from build123d import *

# Parameters (mm, degrees)
SKETCH1_R           = 1.5
BOSS_EXTRUDE1_DEPTH = 3


with BuildPart() as part:
    # Sketch1 → Boss-Extrude1 (new body)
    with BuildSketch(Plane.XY):
        with BuildLine():
            ThreePointArc((-0.4997558, 7.984375), (-0.738146876, 7.96587341), (-0.975878549, 7.94025573))
            ThreePointArc((-0.975878549, 7.94025573), (-1.378121384, 7.372298248), (-1.958371564, 7.756595956))
            ThreePointArc((-1.958371564, 7.756595956), (-2.189303921, 7.694605145), (-2.418280524, 7.625740574))
            ThreePointArc((-2.418280524, 7.625740574), (-2.709312496, 6.993541721), (-3.350297333, 7.264675339))
            ThreePointArc((-3.350297333, 7.264675339), (-3.565906846, 7.161306331), (-3.778330856, 7.05153997))
            ThreePointArc((-3.778330856, 7.05153997), (-3.948241222, 6.376628518), (-4.628132745, 6.525364917))
            ThreePointArc((-4.628132745, 6.525364917), (-4.821077091, 6.384137818), (-5.009714662, 6.237207629))
            ThreePointArc((-5.009714662, 6.237207629), (-5.052717327, 5.542566879), (-5.748362647, 5.563841018))
            ThreePointArc((-5.748362647, 5.563841018), (-5.912071338, 5.389565149), (-6.070498644, 5.210474662))
            ThreePointArc((-6.070498644, 5.210474662), (-5.985129205, 4.519759773), (-6.672838954, 4.412847187))
            ThreePointArc((-6.672838954, 4.412847187), (-6.801737086, 4.211457303), (-6.924559076, 4.006305231))
            ThreePointArc((-6.924559076, 4.006305231), (-6.713724685, 3.343037668), (-7.370079733, 3.111579138))
            ThreePointArc((-7.370079733, 3.111579138), (-7.459777835, 2.889933329), (-7.542811953, 2.66570588))
            ThreePointArc((-7.542811953, 2.66570588), (-7.213692324, 2.052472426), (-7.816341286, 1.704349993))
            ThreePointArc((-7.816341286, 1.704349993), (-7.863784797, 1.469996143), (-7.904203416, 1.234329112))
            ThreePointArc((-7.904203416, 1.234329112), (-7.468006322, 0.692012696), (-7.996426712, 0.239081253))
            ThreePointArc((-7.996426712, 0.239081253), (-8, 0), (-7.996426712, -0.239081253))
            ThreePointArc((-7.996426712, -0.239081253), (-7.468006322, -0.692012696), (-7.904203416, -1.234329112))
            ThreePointArc((-7.904203416, -1.234329112), (-7.863784797, -1.469996143), (-7.816341286, -1.704349993))
            ThreePointArc((-7.816341286, -1.704349993), (-7.213692324, -2.052472426), (-7.542811953, -2.66570588))
            ThreePointArc((-7.542811953, -2.66570588), (-7.459777835, -2.889933329), (-7.370079733, -3.111579138))
            ThreePointArc((-7.370079733, -3.111579138), (-6.713724685, -3.343037668), (-6.924559076, -4.006305231))
            ThreePointArc((-6.924559076, -4.006305231), (-6.801737086, -4.211457303), (-6.672838954, -4.412847187))
            ThreePointArc((-6.672838954, -4.412847187), (-5.985129205, -4.519759773), (-6.070498644, -5.210474662))
            ThreePointArc((-6.070498644, -5.210474662), (-5.912071338, -5.389565149), (-5.748362647, -5.563841018))
            ThreePointArc((-5.748362647, -5.563841018), (-5.052717327, -5.542566879), (-5.009714662, -6.237207629))
            ThreePointArc((-5.009714662, -6.237207629), (-4.821077091, -6.384137818), (-4.628132745, -6.525364917))
            ThreePointArc((-4.628132745, -6.525364917), (-3.948241222, -6.376628518), (-3.778330856, -7.05153997))
            ThreePointArc((-3.778330856, -7.05153997), (-3.565906846, -7.161306331), (-3.350297333, -7.264675339))
            ThreePointArc((-3.350297333, -7.264675339), (-2.709312496, -6.993541721), (-2.418280524, -7.625740574))
            ThreePointArc((-2.418280524, -7.625740574), (-2.189303921, -7.694605145), (-1.958371564, -7.756595956))
            ThreePointArc((-1.958371564, -7.756595956), (-1.378121384, -7.372298248), (-0.975878549, -7.94025573))
            ThreePointArc((-0.975878549, -7.94025573), (-0.738146876, -7.96587341), (-0.4997558, -7.984375))
            ThreePointArc((-0.4997558, -7.984375), (0, -7.5), (0.4997558, -7.984375))
            ThreePointArc((0.4997558, -7.984375), (0.738146876, -7.96587341), (0.975878549, -7.94025573))
            ThreePointArc((0.975878549, -7.94025573), (1.378121384, -7.372298248), (1.958371564, -7.756595956))
            ThreePointArc((1.958371564, -7.756595956), (2.189303921, -7.694605145), (2.418280524, -7.625740574))
            ThreePointArc((2.418280524, -7.625740574), (2.709312496, -6.993541721), (3.350297333, -7.264675339))
            ThreePointArc((3.350297333, -7.264675339), (3.565906846, -7.161306331), (3.778330856, -7.05153997))
            ThreePointArc((3.778330856, -7.05153997), (3.948241222, -6.376628518), (4.628132745, -6.525364917))
            ThreePointArc((4.628132745, -6.525364917), (4.821077091, -6.384137818), (5.009714662, -6.237207629))
            ThreePointArc((5.009714662, -6.237207629), (5.052717327, -5.542566879), (5.748362647, -5.563841018))
            ThreePointArc((5.748362647, -5.563841018), (5.912071338, -5.389565149), (6.070498644, -5.210474662))
            ThreePointArc((6.070498644, -5.210474662), (5.985129205, -4.519759773), (6.672838954, -4.412847187))
            ThreePointArc((6.672838954, -4.412847187), (6.801737086, -4.211457303), (6.924559076, -4.006305231))
            ThreePointArc((6.924559076, -4.006305231), (6.713724685, -3.343037668), (7.370079733, -3.111579138))
            ThreePointArc((7.370079733, -3.111579138), (7.459777835, -2.889933329), (7.542811953, -2.66570588))
            ThreePointArc((7.542811953, -2.66570588), (7.213692324, -2.052472426), (7.816341286, -1.704349993))
            ThreePointArc((7.816341286, -1.704349993), (7.863784797, -1.469996143), (7.904203416, -1.234329112))
            ThreePointArc((7.904203416, -1.234329112), (7.468006322, -0.692012696), (7.996426712, -0.239081253))
            ThreePointArc((7.996426712, -0.239081253), (8, 0), (7.996426712, 0.239081253))
            ThreePointArc((7.996426712, 0.239081253), (7.468006322, 0.692012696), (7.904203416, 1.234329112))
            ThreePointArc((7.904203416, 1.234329112), (7.863784797, 1.469996143), (7.816341286, 1.704349993))
            ThreePointArc((7.816341286, 1.704349993), (7.213692324, 2.052472426), (7.542811953, 2.66570588))
            ThreePointArc((7.542811953, 2.66570588), (7.459777835, 2.889933329), (7.370079733, 3.111579138))
            ThreePointArc((7.370079733, 3.111579138), (6.713724685, 3.343037668), (6.924559076, 4.006305231))
            ThreePointArc((6.924559076, 4.006305231), (6.801737086, 4.211457303), (6.672838954, 4.412847187))
            ThreePointArc((6.672838954, 4.412847187), (5.985129205, 4.519759773), (6.070498644, 5.210474662))
            ThreePointArc((6.070498644, 5.210474662), (5.912071338, 5.389565149), (5.748362647, 5.563841018))
            ThreePointArc((5.748362647, 5.563841018), (5.052717327, 5.542566879), (5.009714662, 6.237207629))
            ThreePointArc((5.009714662, 6.237207629), (4.821077091, 6.384137818), (4.628132745, 6.525364917))
            ThreePointArc((4.628132745, 6.525364917), (3.948241222, 6.376628518), (3.778330856, 7.05153997))
            ThreePointArc((3.778330856, 7.05153997), (3.565906846, 7.161306331), (3.350297333, 7.264675339))
            ThreePointArc((3.350297333, 7.264675339), (2.709312496, 6.993541721), (2.418280524, 7.625740574))
            ThreePointArc((2.418280524, 7.625740574), (2.189303921, 7.694605145), (1.958371564, 7.756595956))
            ThreePointArc((1.958371564, 7.756595956), (1.378121384, 7.372298248), (0.975878549, 7.94025573))
            ThreePointArc((0.975878549, 7.94025573), (0.738146876, 7.96587341), (0.4997558, 7.984375))
            ThreePointArc((0.4997558, 7.984375), (0, 7.5), (-0.4997558, 7.984375))
        make_face()
        Circle(SKETCH1_R, mode=Mode.SUBTRACT)
    extrude(amount=BOSS_EXTRUDE1_DEPTH)


solid = part.part
Can you work these out from the model? Positions are in its coordinate system, mm. Give positions to 0.01 mm unless a question says otherwise; leave off trailing zeros. Loops run counter-clockwise (first coordinate to the right, second up) from the corner with the lowest first, then second, coordinate; pieces in that order, holes last. Notation, with made-up numbers: (66.5, 8) -> (78.5, 8) arc R14 ccw to (78.5, 19) -> close; hole circle Ø1 at (83.25, 41.25). An arc over 180 degrees is marked (long way). Return JSON: item names as keys, results as strings.
Q1. I need wall thicknesses on probe 1 along Y at (x, z) = (0, 1.4); probe 2 along Y at (x, z) = (7.25, 1.9); probe 3 along Y at (x, z) = (-3.5, 2.5). Which ranges of each line are inside material? Lowest first, please.
Checks:
{"probe 1": "y = -7.5 to -1.5, 1.5 to 7.5", "probe 2": "y = -3.07 to -2.42, -1.96 to 1.96, 2.42 to 3.07", "probe 3": "y = -7.19 to 7.19"}
Q2. I want a section at B-B, the plane x = 0. List the corners of the cut face in (y, z) for me.
Checks:
{"outline": "(-7.5, 0) -> (-1.5, 0) -> (-1.5, 3) -> (-7.5, 3) -> close; (1.5, 0) -> (7.5, 0) -> (7.5, 3) -> (1.5, 3) -> close"}
Q3. We'd pull the mould along X, two halves only. Please class faces 1 (the face through (0, -2, 0)), 2 (the face through (5.061, 5.535, 1.479)): released by +X, released by -X, zero draft, split by the parting line, or undercut.
Checks:
{"face 1": "zero draft", "face 2": "undercut"}
Q4. For pin 1 Ø1 at (x, z) = (-4, 1) entering from +Y; pin 2 Ø2.5 at (x, y) = (0, 0) entering from -Z, each with a flat end and sliding along its axis, tell me the tip position at first contact or that it passes through.
Checks:
{"pin 1": "stops at y = 7.19", "pin 2": "passes through"}
Q5. I want a section at A-A, the plane y = 0. List the corners of the cut face in (x, z) for me, then the cut area to 3 significant figures.
Checks:
{"outline": "(-8, 0) -> (-1.5, 0) -> (-1.5, 3) -> (-8, 3) -> close; (1.5, 0) -> (8, 0) -> (8, 3) -> (1.5, 3) -> close", "area": "39.0 mm2"}
Q6. I want a section at C-C, the plane y = -5.75. List the corners of the cut face in (x, z) for me.
Checks:
{"outline": "(-4.92, 0) -> (4.92, 0) -> (4.92, 3) -> (-4.92, 3) -> close"}
